Part model, mm, in its own coordinate system. A direction names the side the tool comes from. Round coordinates to 2 decimals unless told otherwise and drop trailing zeros. Loops run counter-clockwise (first coordinate to the right, second up) from the corner with the lowest first, then second, coordinate; pieces in that order, holes last.
from build123d import *

# Parameters (mm, degrees)
SKETCH2_R           = 4
BOSS_EXTRUDE1_DEPTH = 6.7
SKETCH3_W           = 10
SKETCH3_H           = 13.7
BOSS_EXTRUDE2_DEPTH = 2
SKETCH4_R           = 3.2
CUT_EXTRUDE1_DEPTH  = 6.7
SKETCH7_R           = 1.6
CUT_EXTRUDE4_DEPTH  = 14.956360557
BOSS_EXTRUDE3_START = -8.7
BOSS_EXTRUDE3_DEPTH = 8.7
FILLET2_R           = 2
FILLET3_R           = 3.5


with BuildPart() as part:
    # Sketch2 → Boss-Extrude1 (new body)
    with BuildSketch(Plane(origin=(0, 0, 0), x_dir=(0, 0, -1), z_dir=(1, 0, 0))):
        Circle(SKETCH2_R)
    extrude(amount=-BOSS_EXTRUDE1_DEPTH)

    # Sketch3 → Boss-Extrude2 (add)
    with BuildSketch(Plane.ZY.offset(6.7)):
        with Locations((0, -2.85)):
            Rectangle(SKETCH3_W, SKETCH3_H)
    extrude(amount=BOSS_EXTRUDE2_DEPTH)

    # Sketch4 → Cut-Extrude1 (cut)
    with BuildSketch(Plane(origin=(0, 0, 0), x_dir=(0, 0, -1), z_dir=(1, 0, 0))):
        Circle(SKETCH4_R)
    extrude(amount=-CUT_EXTRUDE1_DEPTH, mode=Mode.SUBTRACT)

    # Sketch7 → Cut-Extrude4 (cut, through all)
    with BuildSketch(Plane.ZY.offset(8.7)):
        Circle(SKETCH7_R)
    extrude(amount=-CUT_EXTRUDE4_DEPTH, mode=Mode.SUBTRACT)

    # Sketch6 → Boss-Extrude3 (add)
    with BuildSketch(Plane.ZY.offset(8.7).offset(BOSS_EXTRUDE3_START)):
        with BuildLine():
            Line((0.7, -2.861817604), (0.7, -2.085665361))
            ThreePointArc((0.7, -2.085665361), (0, -2.2), (-0.7, -2.085665361))
            Line((-0.7, -2.085665361), (-0.7, -2.861817604))
            Line((-0.7, -2.861817604), (-0.7, -3.122498999))
            ThreePointArc((-0.7, -3.122498999), (0, -3.2), (0.7, -3.122498999))
            Line((0.7, -3.122498999), (0.7, -2.861817604))
        make_face()
        with BuildLine():
            Line((-0.7, 2.085665361), (-0.7, 2.861817604))
            Line((-0.7, 2.861817604), (-0.7, 3.122498999))
            ThreePointArc((-0.7, 3.122498999), (0, 3.2), (0.7, 3.122498999))
            Line((0.7, 3.122498999), (0.7, 2.861817604))
            Line((0.7, 2.861817604), (0.7, 2.085665361))
            ThreePointArc((0.7, 2.085665361), (0, 2.2), (-0.7, 2.085665361))
        make_face()
    extrude(amount=BOSS_EXTRUDE3_DEPTH)

    # Fillet2
    fillet2_edges = [part.edges().sort_by_distance(p)[0] for p in [
        (-7.7, 4, -5),
        (-7.7, 4, 5),
    ]]
    fillet(fillet2_edges, radius=FILLET2_R)

    # Fillet3
    fillet3_edges = [part.edges().sort_by_distance(p)[0] for p in [
        (-7.7, -9.7, -5),
        (-7.7, -9.7, 5),
    ]]
    fillet(fillet3_edges, radius=FILLET3_R)


solid = part.part
1) Drop flat-ended pins along their axis: pin 1 Ø2 at (x, y) = (-3.5, -3) entering from +Z; pin 2 Ø0.5 at (x, y) = (-2.5, -2.5) entering from +Z; pin 3 Ø1.1 at (x, y) = (-3.5, -2.5) entering from -Z. Give the stop position or say it passes through.
Values:
pin 1: stops at z = 3.46
pin 2: stops at z = 3.31
pin 3: stops at z = -3.49
2) Slice it at B-B, the plane x = -0.5. Give the cut face in (y, z), then the cut area to 3 significant figures.
Values:
outline: circle Ø8 at (0, 0); hole (-3.12, -0.7) arc R3.2 ccw to (3.12, -0.7) - (2.09, -0.7) arc R2.2 ccw to (2.09, 0.7) - (3.12, 0.7) arc R3.2 ccw to (-3.12, 0.7) - (-2.09, 0.7) arc R2.2 ccw to (-2.09, -0.7) - close
area: 20.9 mm2
3) Slice it at D-D, the plane z = 2.25. Give the cut face in (x, y), then the cut area to 3 significant figures.
Values:
outline: (-8.7, -9.62) - (-6.7, -9.62) - (-6.7, -3.31) - (0, -3.31) - (0, -2.28) - (-6.7, -2.28) - (-6.7, 2.28) - (0, 2.28) - (0, 3.31) - (-6.7, 3.31) - (-6.7, 4) - (-8.7, 4) - close
area: 41.1 mm2
4) Slice it at A-A, the plane y = 0. Give the cut face in (x, z), then the cut area to 3 significant figures.
Values:
outline: (-8.7, -5) - (-6.7, -5) - (-6.7, -4) - (0, -4) - (0, -3.2) - (-6.7, -3.2) - (-6.7, -1.6) - (-8.7, -1.6) - close; (-8.7, 1.6) - (-6.7, 1.6) - (-6.7, 3.2) - (0, 3.2) - (0, 4) - (-6.7, 4) - (-6.7, 5) - (-8.7, 5) - close
area: 24.3 mm2
5) Mould opens along Y. For faces 3 (the face through (-3.3, 2.6, -0.7)), 4 (the face through (-8, -2, -5)), 5 (the face through (-8, 4, 0)), 6 (the face through (-7.71, -8.65, -4)) say: released by +Y, released by -Y, zero draft, split by the parting line, or undercut.
Values:
face 3: undercut
face 4: zero draft
face 5: released by +Y
face 6: released by -Y
6) Slice it at C-C, the plane z = -1. Give the cut face in (x, y), then the cut area to 3 significant figures.
Values:
outline: (-8.7, -9.7) - (-6.7, -9.7) - (-6.7, -3.87) - (0, -3.87) - (0, -3.04) - (-6.7, -3.04) - (-6.7, -1.25) - (-8.7, -1.25) - close; (-8.7, 1.25) - (-6.7, 1.25) - (-6.7, 3.04) - (0, 3.04) - (0, 3.87) - (-6.7, 3.87) - (-6.7, 4) - (-8.7, 4) - close
area: 33.6 mm2
7) Wall check: line 1 along Y through (x, z) = (-2.5, 2); line 2 along X through (y, z) = (0, -4.25); line 3 along Z through (x, y) = (-6, -0.25). Give the ranges that are in metal, low to high.
Values:
line 1: y = -3.46 to -2.5, 2.5 to 3.46
line 2: x = -8.7 to -6.7
line 3: z = -3.99 to -3.19, 3.19 to 3.99
8) Tool access for faces 1 (the face through (-3.3, -2.6, -0.7)), 2 (the face through (-7.71, 3.43, 4.4)): list every direction of +Z, -Z, +X, -X, +Y, -Y with a clear straight run to the whole face (end or side of a thin tool).
Values:
face 1: +X
face 2: +Z, +X, -X, +Y
